```python
from build123d import *

# Parameters (mm, degrees)
SKETCH_R     = 9.5
PAD_DEPTH    = 3
SKETCH002_W  = 9
SKETCH002_H  = 9
PAD001_DEPTH = 21
CHAMFER_SIZE = 1
SKETCH003_R  = 1.75
POCKET_DEPTH = 21


with BuildPart() as part:
    # Sketch → Pad (new body)
    with BuildSketch(Plane.XY):
        Circle(SKETCH_R)
    extrude(amount=PAD_DEPTH)

    # Sketch002 (on Face3 of Pad) → Pad001 (join)
    with BuildSketch(Plane.XY.offset(3)):
        Rectangle(SKETCH002_W, SKETCH002_H)
    extrude(amount=PAD001_DEPTH)

    # Chamfer
    chamfer_edges = [part.edges().sort_by_distance(p)[0] for p in [
        (0, 4.5, 24),
        (-4.5, 0, 24),
        (0, -4.5, 24),
        (4.5, 0, 24),
    ]]
    chamfer(chamfer_edges, length=CHAMFER_SIZE)

    # Sketch003 (on Face8 of Chamfer) → Pocket (cut)
    with BuildSketch(Plane.XY.offset(24)):
        with Locations((0.020416, -0.031336)):
            Circle(SKETCH003_R)
    extrude(amount=-POCKET_DEPTH, mode=Mode.SUBTRACT)


solid = part.part
```
Geometry check sheet. Reference: the model listing, model coordinates, mm. A direction names the side the tool comes from. Coordinates: 2 decimals unless noted, no trailing zeros. Write each loop counter-clockwise with the first axis right and the second up, starting at its lowest first coordinate (ties: lowest second). Pieces come first, ordered by that corner, then holes. Notation, with made-up numbers: M 55,28 L 108,28 A18 ccw 108,59 Z; hole C 24.25,70.5 d9. An arc over 180 degrees is marked long. One line per item, written item: value. Start each with the question number.
(1) Sectioned sample at B-B, the plane z = 16.5. Enter the section's corners in (x, y).
(2) Sectioned sample at C-C, the plane y = -6. Enter the section's corners in (x, z), and give its area (3 significant figures).
(3) Tool access check on faces 1 (the face through (-4.5, 0, 13)), 2 (the face through (-1.728, 0.046, 13.647)), 3 (the face through (0, 4.5, 13)), 4 (the face through (0, 0, 0)), 5 (the face through (4, -0.1, 23.5)). Record the directions out of +Z, -Z, +X, -X, +Y, -Y that give a thin tool (end or side, any length) a straight path to the whole face; none if there is none.
(4) Scan lines: line 1 along Z through (x, y) = (8.25, 2.5); line 2 along Y through (x, z) = (-2, 20). Record each from-to range of solid material in increasing order. Write a range as [from, to].
(5) Sectioned sample at A-A, the plane x = 0. Enter the section's corners in (y, z), and give its area (3 significant figures).
(6) Release check for a two-part mould opening along Y. For faces 6 (the face through (0, 0, 3)), 7 (the face through (4.5, 0, 13)), 8 (the face through (-0.1, 4, 23.5)), 9 (the face through (0, -4.5, 13)) record: released by +Y, released by -Y, zero draft, split by the parting line, or undercut.
(7) Sectioned sample at D-D, the plane x = 7.5. Enter the section's corners in (y, z).
(8) Depth check by flat-ended pin: pin 1 (10 mm diameter, centred on x = -1, z = 12, fed in from +Y); pin 2 (5 mm diameter, centred on y = 1.5, z = 19, fed in from -X); pin 3 (2.5 mm diameter, centred on x = 1, z = 11.5, fed in from -Y). Enter the tip coordinate at first touch or a pass-through.
Filled sheet:
1. outline: M -4.5,-4.5 L 4.5,-4.5 L 4.5,4.5 L -4.5,4.5 Z; hole C 0.02,-0.03 d3.5
2. outline: M -7.37,0 L 7.37,0 L 7.37,3 L -7.37,3 Z
2. area: 44.2 mm²
3. face 1: +Z, -X, +Y, -Y
3. face 2: +Z
3. face 3: +Z, +X, -X, +Y
3. face 4: -Z, +X, -X, +Y, -Y
3. face 5: +Z, +X, +Y, -Y
4. line 1: [0, 3]
4. line 2: [-4.5, 4.5]
5. outline: M -9.5,0 L 9.5,0 L 9.5,3 L 4.5,3 L 4.5,23 L 3.5,24 L 1.72,24 L 1.72,3 L -1.78,3 L -1.78,24 L -3.5,24 L -4.5,23 L -4.5,3 L -9.5,3 Z
5. area: 172 mm²
6. face 6: undercut
6. face 7: zero draft
6. face 8: released by +Y
6. face 9: released by -Y
7. outline: M -5.83,0 L 5.83,0 L 5.83,3 L -5.83,3 Z
8. pin 1: y = 4.5
8. pin 2: x = -4.5
8. pin 3: y = -4.5
